```python
from build123d import *


with BuildPart() as part:
    # Schizzo1 → Rivoluzione1 (revolve)
    with BuildSketch(Plane(origin=(0, 0, 0), x_dir=(0, 0, -1), z_dir=(1, 0, 0))):
        Polygon((-100, 180), (-95, 180), (-81.602540378, 130), (-6.113497125, 0), (-6.113497125, -2), (-4.25, -2), (-4.25, 0), (-79.739043254, 130), (-93.261333513, 180.465874281), (-96.887791569, 194), (-101.8, 194), (-101.8, 170), (-100, 170), align=None)
    revolve(axis=Axis((0, 0, 0), (0, 1, 0)))


solid = part.part
```
The listing builds one solid part. Answer for the finished solid, in the listing's coordinates (mm). A direction names the side the tool comes from. Coordinates: 2 decimals unless noted, no trailing zeros. Write each loop counter-clockwise with the first axis right and the second up, starting at its lowest first coordinate (ties: lowest second). Pieces come first, ordered by that corner, then holes. Notation, with made-up numbers: M 29.25,82 L 63.25,82 A35 cw 63.25,119 Z; hole C -3.75,44 d11. An arc over 180 degrees is marked long. Use a Markdown table: item, result. Add a question column.
1. For a pull along Z with two mould halves and no side action, classify faces 3 (the cylindrical face through (85.838, 181.832, 54.727)), 4 (the cylindrical face through (30.04, 175.07, 95.38)), 5 (the flat face through (-67, 170, 75)) as +Z half, -Z half, draft (parallel to the pull), parting line (faces both ways), or undercut.
2. Given P1, Ø6, axis at x = -60.5, y = 85, coming from the -Z side; P2, Ø2, axis at y = 87.5, z = 11, coming from the +X side; P3, Ø1, axis at x = 8, z = 4.5, coming from the -Y side; P4, Ø12, axis at y = 171.5, z = 27, coming from the +X side, each flat-ended and moving along its own axis, determine where each tip first touches the part or whether it passes through.
3. Which of the six approach directions +Z, -Z, +X, -X, +Y, -Y give full straight-line access (tool end or side, diameter ignored) to faces 1 (the flat face through (-37, 180, 88)), 2 (the flat face through (-37, 194, -90))?
4. Straight lines are drawn through the part: line 1 along X through (y, z) = (0, 0); line 2 along X through (y, z) = (176, 0); line 3 along X through (y, z) = (174.75, 0). For each, find the intervals that lie inside material, in ascending order. Write a range as [from, to].
5. Section B-B (y = 125) is taken. Give the vertices of the cut face in (x, z).
6. Section A-A (y = 100.5) is taken. Give the vertices of the cut face in (x, z), plus the area to 3 significant figures.
Data:
| question | item | result |
|---|---|---|
| 1 | face 3 | parting line |
| 1 | face 4 | undercut |
| 1 | face 5 | draft |
| 2 | P1 | passes through |
| 2 | P2 | stops at x = 56.47 |
| 2 | P3 | stops at y = 4.42 |
| 2 | P4 | stops at x = 99.61 |
| 3 | face 1 | -Y |
| 3 | face 2 | +Z, -Z, +X, -X, +Y |
| 4 | line 1 | x = [-6.11, -4.25], [4.25, 6.11] |
| 4 | line 2 | x = [-101.8, -100], [-93.93, -92.06], [92.06, 93.93], [100, 101.8] |
| 4 | line 3 | x = [-101.8, -100], [-93.59, -91.73], [91.73, 93.59], [100, 101.8] |
| 5 | outline | C 0,0 d157.4; hole C 0,0 d153.67 |
| 6 | outline | C 0,0 d128.94; hole C 0,0 d125.22 |
| 6 | area | 744 mm2 |
